```python
from build123d import *
from OCP.BRepFilletAPI import BRepFilletAPI_MakeFillet

# Parameters (mm, degrees)
BOSS_EXTRUDE1_DEPTH = 3.175
SKETCH3_R           = 2.032
CUT_EXTRUDE1_DEPTH  = 241.986473946
FILLET1_R           = 6.35
SKETCH4_R           = 2.032
SKETCH4_W           = 19.05
SKETCH4_H           = 29.448186152
CUT_EXTRUDE2_DEPTH  = 241.986473946
FILLET2_R           = 12.7
FILLET2_R_2         = 6.35


with BuildPart() as part:
    # Sketch1 → Boss-Extrude1 (new body)
    with BuildSketch(Plane(origin=(0, 0, 0), x_dir=(1, 0, 0), z_dir=(0, 1, 0))):
        with BuildLine():
            Line((0, 0), (0, 76.2))
            Line((0, 76.2), (228.6, 76.2))
            Line((228.6, 76.2), (228.6, 0))
            ThreePointArc((228.6, 0), (114.3, 57.15), (0, 0))
        make_face()
    extrude(amount=BOSS_EXTRUDE1_DEPTH)

    # Sketch3 → Cut-Extrude1 (cut, through all)
    with BuildSketch(Plane.XZ):
        with Locations(Location((36.5125, -49.2125, 0), (0, 0, 270))):
            Circle(SKETCH3_R)
        with Locations(Location((26.9875, -49.2125, 0), (0, 0, 270))):
            Circle(SKETCH3_R)
        with Locations(Location((201.6125, -49.2125, 0), (0, 0, 90))):
            Circle(SKETCH3_R)
        with Locations(Location((192.0875, -49.2125, 0), (0, 0, 90))):
            Circle(SKETCH3_R)
        with Locations(Location((36.5125, -71.4375, 0), (0, 0, 270))):
            Circle(SKETCH3_R)
        with Locations(Location((26.9875, -71.4375, 0), (0, 0, 270))):
            Circle(SKETCH3_R)
        with Locations(Location((201.6125, -71.4375, 0), (0, 0, 90))):
            Circle(SKETCH3_R)
        with Locations(Location((192.0875, -71.4375, 0), (0, 0, 90))):
            Circle(SKETCH3_R)
    extrude(amount=-CUT_EXTRUDE1_DEPTH, mode=Mode.SUBTRACT)

    # Fillet1
    fillet1_edges = [part.edges().sort_by_distance(p)[0] for p in [
        (0, 1.5875, 0),
        (228.6, 1.5875, 0),
    ]]
    fillet(fillet1_edges, radius=FILLET1_R)

    # Sketch4 → Cut-Extrude2 (cut, through all)
    with BuildSketch(Plane.XZ):
        with Locations(Location((6.35, -17.303627696, 0), (0, 0, 270))):
            Circle(SKETCH4_R)
        with Locations(Location((6.35, -30.003627696, 0), (0, 0, 270))):
            Circle(SKETCH4_R)
        with Locations(Location((222.25, -17.303627696, 0), (0, 0, 270))):
            Circle(SKETCH4_R)
        with Locations(Location((222.25, -30.003627696, 0), (0, 0, 270))):
            Circle(SKETCH4_R)
        with Locations((9.525, -61.475906924)):
            Rectangle(SKETCH4_W, SKETCH4_H)
        with Locations((219.075, -61.475906924)):
            Rectangle(SKETCH4_W, SKETCH4_H)
    extrude(amount=-CUT_EXTRUDE2_DEPTH, mode=Mode.SUBTRACT)

    # Fillet2
    fillet2_edges_1 = [part.edges().sort_by_distance(p)[0] for p in [
        (209.55, 1.5875, -46.751813848),
        (19.05, 1.5875, -46.751813848),
    ]]
    fillet2_edges_2 = [part.edges().sort_by_distance(p)[0] for p in [
        (228.6, 1.5875, -46.751813848),
        (209.55, 1.5875, -76.2),
        (0, 1.5875, -46.751813848),
        (19.05, 1.5875, -76.2),
    ]]
    fillet2 = BRepFilletAPI_MakeFillet(part.part.solid().wrapped)
    for e in fillet2_edges_1:
        fillet2.Add(FILLET2_R - 0.0001, e.wrapped)
    for e in fillet2_edges_2:
        fillet2.Add(FILLET2_R_2 - 0.0001, e.wrapped)
    add(Compound.cast(fillet2.Shape()), mode=Mode.REPLACE)  # a hair under: the kernel refuses the full size


solid = part.part
```
Design review of the part built by this model. Coordinates are the model's own, in mm. Give positions to 0.01 mm unless a question says otherwise; leave off trailing zeros. Write each loop counter-clockwise with the first axis right and the second up, starting at its lowest first coordinate (ties: lowest second). Pieces come first, ordered by that corner, then holes. Notation, with made-up numbers: (68.25, 65.5) -> (124.25, 65.5) arc R34 cw to (124.25, 101.5) -> close; hole circle Ø10 at (28, 58.5). An arc over 180 degrees is marked (long way). Answer in a Markdown table with one row per item.
(1) Consider section C-C (z = -63). State the section outline as (x, y) points (3 decimals).
Results:
| item | result |
|---|---|
| outline | (19.05, 0) -> (209.55, 0) -> (209.55, 3.175) -> (19.05, 3.175) -> close |
(2) To check wall thickness, follow probe 1 along X at (y, z) = (2.9, -15.5); probe 2 along Z at (x, y) = (222.25, 2.45); probe 3 along Z at (x, y) = (202, 1.4). State the ranges of each line that lie inside material, in increasing order.
Results:
| item | result |
|---|---|
| probe 1 | 0.26 to 5.41, 7.29 to 13.47, 215.13 to 221.31, 223.19 to 228.34 |
| probe 2 | -46.75 to -32.04, -27.97 to -19.34, -15.27 to -10.95 |
| probe 3 | -76.2 to -73.43, -69.44 to -51.21, -47.22 to -27.07 |
(3) Consider section A-A (z = -35.5). State the section outline as (x, y) points (3 decimals), then the cut area to 3 significant figures.
Results:
| item | result |
|---|---|
| outline | (0, 0) -> (38.684, 0) -> (38.684, 3.175) -> (0, 3.175) -> close; (189.916, 0) -> (228.6, 0) -> (228.6, 3.175) -> (189.916, 3.175) -> close |
| area | 246 mm2 |
(4) Consider section B-B (y = 1.85). Count the separate pieces of the cut face and the enclosed holes in it, then the cut area to 3 significant figures.
Results:
| item | result |
|---|---|
| separate pieces | 1 |
| enclosed holes | 12 |
| area | 6,930 mm2 |
(5) Mouldability with a two-part tool opening along Z and no side actions: class faces 1 (the cylindrical face through (193.32, 1.57, -50.83)), 2 (the cylindrical face through (15.23, 1.61, -50.37)), 3 (the cylindrical face through (25.004, 1.565, -70.997)), 4 (the cylindrical face through (115.92, 1.57, -57.14)) as +Z half, -Z half, draft (parallel to the pull), parting line (faces both ways), or undercut.
Results:
| item | result |
|---|---|
| face 1 | undercut |
| face 2 | -Z half |
| face 3 | undercut |
| face 4 | +Z half |
(6) Consider section D-D (x = 170). State the section outline as (y, z) points (3 decimals).
Results:
| item | result |
|---|---|
| outline | (0, -76.2) -> (3.175, -76.2) -> (3.175, -45.845) -> (0, -45.845) -> close |
(7) Clearance check with a flat-ended pin moving along its axis: pin 1 (1.6 mm diameter, centred on y = 2.5, z = -65, fed in from -X). State where the tip first meets the part, or that it passes through.
Results:
| item | result |
|---|---|
| pin 1 | x = 19.05 |
